```python
from build123d import *

# Parameters (mm, degrees)
SKETCH1_W           = 241
SKETCH1_H           = 374
BOSS_EXTRUDE1_DEPTH = 20
SKETCH5_R           = 8.426003706
BOSS_EXTRUDE3_DEPTH = 20
SKETCH6_W           = 241
SKETCH6_H           = 20
CUT_EXTRUDE1_DEPTH  = 5
SKETCH7_R           = 8.40478741
BOSS_EXTRUDE4_DEPTH = 20
SKETCH8_W           = 20
SKETCH8_H           = 369
CUT_EXTRUDE2_DEPTH  = 5
SKETCH9_W           = 20
SKETCH9_H           = 369
CUT_EXTRUDE3_DEPTH  = 5
SKETCH11_R          = 8.426003706
CUT_EXTRUDE4_DEPTH  = 10
SKETCH12_R          = 8.40478741
CUT_EXTRUDE5_DEPTH  = 10
SKETCH13_R          = 8.40478741
BOSS_EXTRUDE6_DEPTH = 10
SKETCH14_R          = 8.426003706
BOSS_EXTRUDE7_DEPTH = 10
SKETCH15_W          = 231
SKETCH15_H          = 20
CUT_EXTRUDE6_DEPTH  = 5
SKETCH16_R          = 8.05
BOSS_EXTRUDE8_DEPTH = 20


with BuildPart() as part:
    # Sketch1 → Boss-Extrude1 (new body)
    with BuildSketch(Plane.XY):
        with Locations((93.728999485, -168.226086957)):
            Rectangle(SKETCH1_W, SKETCH1_H)
    extrude(amount=BOSS_EXTRUDE1_DEPTH)

    # Sketch5 → Boss-Extrude3 (add)
    with BuildSketch(Plane.XZ.offset(355.226086957)):
        with Locations(Location((93.728999485, 10.577560917, 0), (0, 0, 90))):
            Circle(SKETCH5_R)
    extrude(amount=BOSS_EXTRUDE3_DEPTH)

    # Sketch6 → Cut-Extrude1 (cut)
    with BuildSketch(Plane(origin=(0, 18.773913043, 0), x_dir=(1, 0, 0), z_dir=(0, 1, 0))):
        with Locations((93.728999485, -10)):
            Rectangle(SKETCH6_W, SKETCH6_H)
    extrude(amount=-CUT_EXTRUDE1_DEPTH, mode=Mode.SUBTRACT)

    # Sketch7 → Boss-Extrude4 (add)
    with BuildSketch(Plane(origin=(0, 13.773913043, 0), x_dir=(1, 0, 0), z_dir=(0, 1, 0))):
        with Locations(Location((93.728999485, -10.486825902, 0), (0, 0, 270))):
            Circle(SKETCH7_R)
    extrude(amount=BOSS_EXTRUDE4_DEPTH)

    # Sketch8 → Cut-Extrude2 (cut)
    with BuildSketch(Plane.ZY.offset(26.771000515)):
        with Locations((10, -170.726086957)):
            Rectangle(SKETCH8_W, SKETCH8_H)
    extrude(amount=-CUT_EXTRUDE2_DEPTH, mode=Mode.SUBTRACT)

    # Sketch9 → Cut-Extrude3 (cut)
    with BuildSketch(Plane(origin=(214.228999485, 0, 0), x_dir=(0, 0, -1), z_dir=(1, 0, 0))):
        with Locations((-10, -170.726086957)):
            Rectangle(SKETCH9_W, SKETCH9_H)
    extrude(amount=-CUT_EXTRUDE3_DEPTH, mode=Mode.SUBTRACT)

    # Sketch11 → Cut-Extrude4 (cut)
    with BuildSketch(Plane.XZ.offset(375.226086957)):
        with Locations(Location((93.728999485, 10.577560917, 0), (0, 0, 90))):
            Circle(SKETCH11_R)
    extrude(amount=-CUT_EXTRUDE4_DEPTH, mode=Mode.SUBTRACT)

    # Sketch12 → Cut-Extrude5 (cut)
    with BuildSketch(Plane(origin=(0, 33.773913043, 0), x_dir=(1, 0, 0), z_dir=(0, 1, 0))):
        with Locations(Location((93.728999485, -10.486825902, 0), (0, 0, 270))):
            Circle(SKETCH12_R)
    extrude(amount=-CUT_EXTRUDE5_DEPTH, mode=Mode.SUBTRACT)

    # Sketch13 → Boss-Extrude6 (add)
    with BuildSketch(Plane(origin=(0, 23.773913043, 0), x_dir=(1, 0, 0), z_dir=(0, 1, 0))):
        with Locations(Location((93.728999485, -10.486825902, 0), (0, 0, 270))):
            Circle(SKETCH13_R)
    extrude(amount=BOSS_EXTRUDE6_DEPTH)

    # Sketch14 → Boss-Extrude7 (add)
    with BuildSketch(Plane.XZ.offset(365.226086957)):
        with Locations(Location((93.728999485, 10.577560917, 0), (0, 0, 90))):
            Circle(SKETCH14_R)
    extrude(amount=BOSS_EXTRUDE7_DEPTH)

    # Sketch15 → Cut-Extrude6 (cut)
    with BuildSketch(Plane(origin=(0, 13.773913043, 0), x_dir=(1, 0, 0), z_dir=(0, 1, 0))):
        with Locations((93.728999485, -10)):
            Rectangle(SKETCH15_W, SKETCH15_H)
    extrude(amount=-CUT_EXTRUDE6_DEPTH, mode=Mode.SUBTRACT)


with BuildPart() as body_2:
    # of the pieces the cut leaves, the one that is kept (cut_extrude6_keep)
    add(part.part.solids().sort_by_distance((-21.771000515, 8.773913043, 0))[0])

    # Sketch16 → Boss-Extrude8 (add)
    with BuildSketch(Plane(origin=(0, 8.773913043, 0), x_dir=(1, 0, 0), z_dir=(0, 1, 0))):
        with Locations(Location((93.728999485, -10.577560917, 0), (0, 0, 270))):
            Circle(SKETCH16_R)
    extrude(amount=BOSS_EXTRUDE8_DEPTH)


solid = body_2.part
```
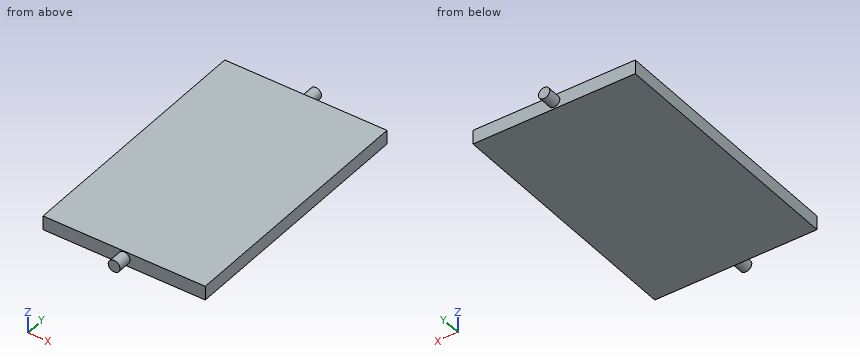
Geometry check sheet. Reference: the model listing, model coordinates, mm. Coordinates: 2 decimals unless noted, no trailing zeros. Order: outer loops, then holes, each group sorted by start corner. A loop starts at its lowest first (then second) coordinate and runs counter-clockwise, first axis right, second up.
Item 1: Section check B-B (z = 14.5). Enter the section's corners in (x, y), plus the area to 3 significant figures.
Item 2: Depth check by flat-ended pin: pin 1 (1 mm diameter, centred on x = 131.5, z = 3.5, fed in from -Y); pin 2 (10 mm diameter, centred on x = 80.5, z = 4.5, fed in from +Y); pin 3 (6 mm diameter, centred on x = 102, z = 6.5, fed in from +Y). Enter the tip coordinate at first touch or a pass-through.
Item 3: Section check A-A (x = 26.5). Enter the section's corners in (y, z).
Item 4: Scan lines: line 1 along Y through (x, z) = (141, 13.25); line 2 along Y through (x, z) = (98, 3.5). Record each from-to range of solid material in increasing order.
Check sheet entries:
1. outline: (-21.77, -355.23) - (86.27, -355.23) - (86.27, -375.23) - (101.19, -375.23) - (101.19, -355.23) - (209.23, -355.23) - (209.23, 8.77) - (100.76, 8.77) - (100.76, 28.77) - (86.7, 28.77) - (86.7, 8.77) - (-21.77, 8.77) - close
1. area: 84,700 mm2
2. pin 1: stops at y = -355.23
2. pin 2: stops at y = 8.77
2. pin 3: stops at y = 28.77
3. outline: (-355.23, 0) - (8.77, 0) - (8.77, 20) - (-355.23, 20) - close
4. line 1: y = -355.23 to 8.77
4. line 2: y = -375.23 to 8.77
